Drawing for the job (mm, zero at the part's lowest x, y, z). A direction names the side the tool comes from. Round coordinates to 2 decimals unless told otherwise and drop trailing zeros. Write each loop counter-clockwise with the first axis right and the second up, starting at its lowest first coordinate (ties: lowest second). Pieces come first, ordered by that corner, then holes.
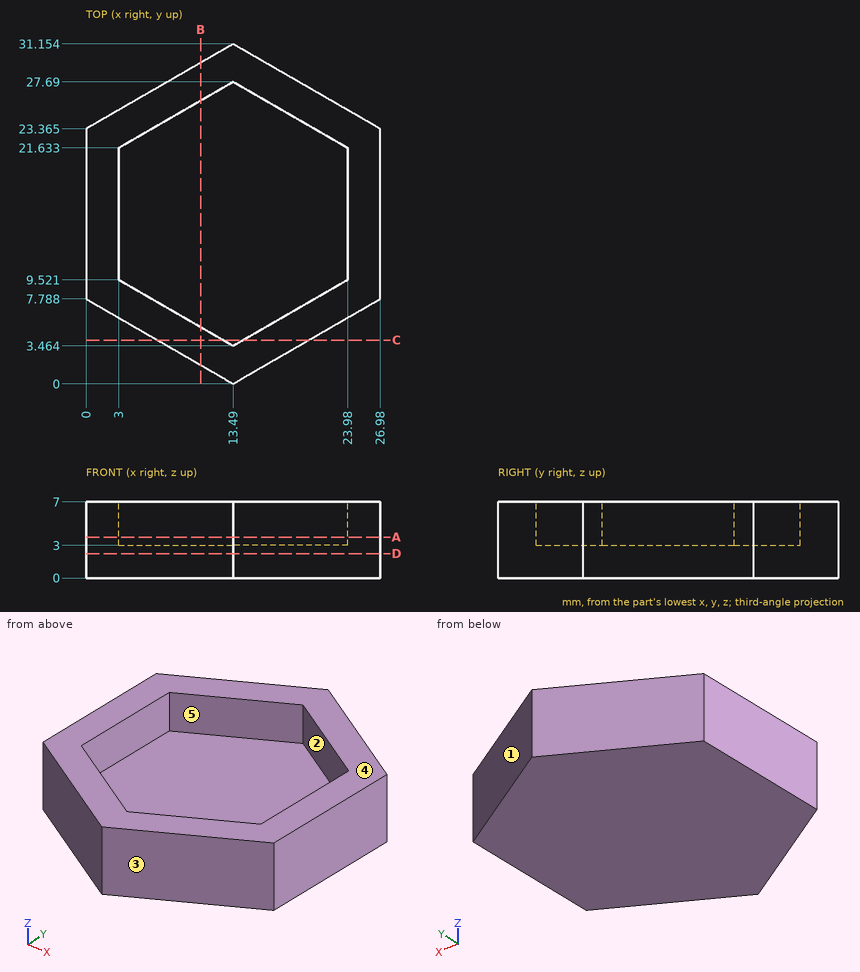
Q1. Saw through at C-C, the plane y = 4. Write the cut outline in (x, z).
Q2. Drop flat-ended pins along their axis: P1, Ø3, axis at x = 24, z = 3.5, coming from the +Y side; P2, Ø3, axis at x = 23, z = 5, coming from the -Y side (1 decimal); P3, Ø2, axis at x = 5, z = 6, coming from the +Y side. Give the stop position or say it passes through.
Q3. Saw through at B-B, the plane x = 10.5. Write the cut outline in (y, z), and give its area (3 significant figures).
Q4. Saw through at A-A, the plane z = 3.75. Write the cut outline in (x, y) (1 decimal).
Q5. Wall check: line 1 (X direction, y = 20, z = 6.5); line 2 (Z direction, x = 7.25, y = 21); line 3 (Y direction, x = 14.5, z = 3.5) (1 decimal). Give the ranges that are in metal, low to high.
Q6. Saw through at D-D, the plane z = 2.25. Write the cut outline in (x, y) (1 decimal), and give its area (3 significant figures).
Q7. Two-plate mould, pull along X, no slides. Class the marked faces 3, 4 and 5: released by +X, released by -X, zero draft, split by the parting line, or undercut.
Q8. Tool access for the marked faces 1 and 2: list every direction of +Z, -Z, +X, -X, +Y, -Y with a clear straight run to the whole face (end or side of a thin tool).
Computed:
1. outline: (6.56, 0) - (20.42, 0) - (20.42, 7) - (14.42, 7) - (14.42, 3) - (12.56, 3) - (12.56, 7) - (6.56, 7) - close
2. P1: stops at y = 25.95
2. P2: stops at y = 4.6
2. P3: stops at y = 26.83
3. outline: (1.73, 0) - (29.43, 0) - (29.43, 7) - (25.96, 7) - (25.96, 3) - (5.19, 3) - (5.19, 7) - (1.73, 7) - close
3. area: 111 mm2
4. outline: (0, 7.8) - (13.5, 0) - (27, 7.8) - (27, 23.4) - (13.5, 31.2) - (0, 23.4) - close; hole (3, 9.5) - (13.5, 3.5) - (24, 9.5) - (24, 21.6) - (13.5, 27.7) - (3, 21.6) - close
5. line 1: x = 0 to 3, 23.98 to 26.98
5. line 2: z = 0 to 3
5. line 3: y = 0.6 to 4, 27.1 to 30.6
6. outline: (0, 7.8) - (13.5, 0) - (27, 7.8) - (27, 23.4) - (13.5, 31.2) - (0, 23.4) - close
6. area: 630 mm2
7. face 3: released by +X
7. face 4: zero draft
7. face 5: undercut
8. face 1: +Z, -Z, +X, +Y
8. face 2: +Z
